The model under review builds one solid part; all positions refer to its coordinate system, in mm. Face numbers are marked on the shaded views. A direction names the side the tool comes from. Give positions to 0.01 mm unless a question says otherwise; leave off trailing zeros. Write each loop counter-clockwise with the first axis right and the second up, starting at its lowest first coordinate (ties: lowest second). Pieces come first, ordered by that corner, then holes. Notation, with made-up numbers: (18.5, -14) -> (65.5, -14) arc R13 cw to (65.5, -3) -> close; hole circle Ø6 at (53, 58). An arc over 180 degrees is marked (long way). Use CSV: the item, a comma, the result in double quotes.
```python
from build123d import *

# Parameters (mm, degrees)
SKETCH_W        = 37
SKETCH_H        = 32
PAD_DEPTH       = 4
SKETCH001_W     = 4
SKETCH001_H     = 32
PAD001_DEPTH    = 10
SKETCH002_R     = 1.4
POCKET_DEPTH    = 100
POCKET003_DEPTH = 100
SKETCH004_R     = 1.3
SKETCH004_R_2   = 4.5
POCKET007_DEPTH = 5
SKETCH008_R     = 1.8
POCKET009_DEPTH = 10
CHAMFER_SIZE    = 1
CHAMFER001_SIZE = 0.2


with BuildPart() as part:
    # Sketch → Pad (new body)
    with BuildSketch(Plane.XY):
        Rectangle(SKETCH_W, SKETCH_H)
    extrude(amount=PAD_DEPTH)

    # Sketch001 (on Face6 of Pad) → Pad001 (join)
    with BuildSketch(Plane.XY.offset(4)):
        with Locations((16.5, 0)):
            Rectangle(SKETCH001_W, SKETCH001_H)
        with Locations((-16.5, 0)):
            Rectangle(SKETCH001_W, SKETCH001_H)
    extrude(amount=PAD001_DEPTH)

    # Sketch002 (on Face13 of Pad001) → Pocket (cut)
    with BuildSketch(Plane.YZ.offset(18.5)):
        with Locations((-11, 11)):
            Circle(SKETCH002_R)
        with Locations((11, 11)):
            Circle(SKETCH002_R)
    extrude(amount=-POCKET_DEPTH, mode=Mode.SUBTRACT)

    # Sketch006 → Pocket003 (cut)
    with BuildSketch(Plane(origin=(-20, 0, 0), x_dir=(0, -1, 0), z_dir=(-1, 0, 0))):
        with BuildLine():
            ThreePointArc((8, 10.650166), (0, 29.2), (-8, 10.650166))
            Line((-8, 10.650166), (-8, 7.2))
            Line((-8, 7.2), (8, 7.2))
            Line((8, 7.2), (8, 10.650166))
        make_face()
    extrude(amount=-POCKET003_DEPTH, mode=Mode.SUBTRACT)

    # Sketch004 → Pocket007 (cut)
    with BuildSketch(Plane.XY.offset(4)):
        with Locations((0, 8)):
            Circle(SKETCH004_R)
        with Locations((8, 0)):
            Circle(SKETCH004_R)
        with Locations((0, -8)):
            Circle(SKETCH004_R)
        with Locations((-8, 0)):
            Circle(SKETCH004_R)
        Circle(SKETCH004_R_2)
        with Locations((5.656854, 5.656854)):
            Circle(SKETCH004_R)
        with Locations((-5.656854, 5.656854)):
            Circle(SKETCH004_R)
        with Locations((-5.656854, -5.656854)):
            Circle(SKETCH004_R)
        with Locations((5.656854, -5.656854)):
            Circle(SKETCH004_R)
    extrude(amount=-POCKET007_DEPTH, mode=Mode.SUBTRACT)

    # Sketch008 → Pocket009 (cut)
    with BuildSketch(Plane(origin=(0, 0, 0), x_dir=(1, 0, 0), z_dir=(0, 0, -1))):
        with Locations((10, 10)):
            Circle(SKETCH008_R)
        with Locations((-10, 10)):
            Circle(SKETCH008_R)
        with Locations((-10, -10)):
            Circle(SKETCH008_R)
        with Locations((10, -10)):
            Circle(SKETCH008_R)
    extrude(amount=-POCKET009_DEPTH, mode=Mode.SUBTRACT)

    # Chamfer
    chamfer_edges = [part.edges().sort_by_distance(p)[0] for p in [
        (-6.956854, -5.656854, 4),
        (-1.3, -8, 4),
        (4.356854, -5.656854, 4),
        (6.7, 0, 4),
        (4.356854, 5.656854, 4),
        (-1.3, 8, 4),
        (-6.956854, 5.656854, 4),
        (-9.3, 0, 4),
    ]]
    chamfer(chamfer_edges, length=CHAMFER_SIZE)

    # Chamfer001
    chamfer001_edges = [part.edges().sort_by_distance(p)[0] for p in [
        (-6.956854, -5.656854, 0),
        (-9.3, 0, 0),
        (-6.956854, 5.656854, 0),
        (-1.3, 8, 0),
        (4.356854, 5.656854, 0),
        (6.7, 0, 0),
        (4.356854, -5.656854, 0),
        (-1.3, -8, 0),
        (-11.8, -10, 0),
        (-11.8, 10, 0),
        (8.2, 10, 0),
        (8.2, -10, 0),
    ]]
    chamfer(chamfer001_edges, length=CHAMFER001_SIZE)


solid = part.part
```
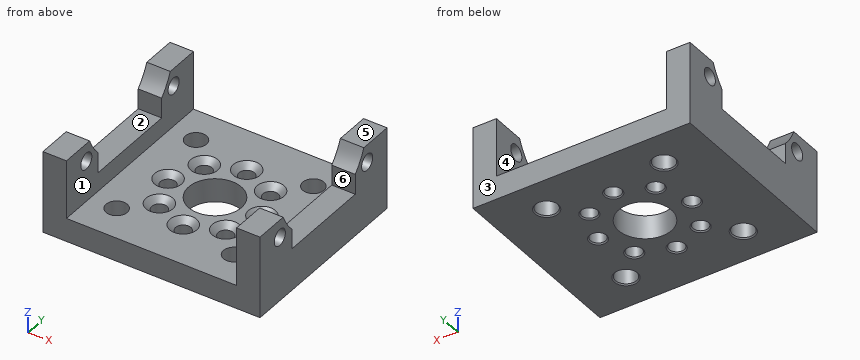
Q1. The part is to be moulded in two halves that separate along Y. For the marked faces 1, 2 and 3, say which applies: pulls with the +Y half, pulls with the -Y half, needs draft (parallel to the pull), parting line crosses it, or undercut.
Derived:
face 1,"needs draft"
face 2,"undercut"
face 3,"pulls with the +Y half"
Q2. Consider section B-B (x = 0). Write out the cut boundary in (y, z), then the cut area to 3 significant figures.
Derived:
outline,"(-16, 0) -> (-9.5, 0) -> (-9.3, 0.2) -> (-9.3, 3) -> (-10.3, 4) -> (-16, 4) -> close; (-6.7, 0.2) -> (-6.5, 0) -> (-4.5, 0) -> (-4.5, 4) -> (-5.7, 4) -> (-6.7, 3) -> close; (4.5, 0) -> (6.5, 0) -> (6.7, 0.2) -> (6.7, 3) -> (5.7, 4) -> (4.5, 4) -> close; (9.3, 0.2) -> (9.5, 0) -> (16, 0) -> (16, 4) -> (10.3, 4) -> (9.3, 3) -> close"
area,"69.1 mm2"
Q3. Machinability: for the marked faces 4, 5 and 6, which of the approach directions +Z, -Z, +X, -X, +Y, -Y give a long, thin tool a straight path to every point of the face, cutting with its end or side? Answer none if there is none.
Derived:
face 4,"+Z, +Y, -Y"
face 5,"+Z, +X, -X, +Y, -Y"
face 6,"+Z, +X, -X"
Q4. Insertion check: pin 1 (3.5 mm diameter, centred on x = -5.66, y = -5.66, fed in from -Z); pin 2 (4 mm diameter, centred on x = -10, y = -10, fed in from +Z); pin 3 (2 mm diameter, centred on x = -8, y = 0, fed in from -Z); pin 4 (3 mm diameter, centred on x = 0, y = 8, fed in from +Z). Each pin has a flat end and moves straight along its axis. Give the tip position at first contact, or say it passes through.
Derived:
pin 1,"stops at z = 0"
pin 2,"stops at z = 4"
pin 3,"passes through"
pin 4,"stops at z = 3.2"
Q5. Consider section C-C (z = 2). State how many separate pieces and enclosed holes the cut face has, then the cut area to 3 significant figures.
Derived:
separate pieces,"1"
enclosed holes,"13"
area,"1,040 mm2"
Q6. To check wall thickness, follow probe 1 along X at (y, z) = (-10, 3.2); probe 2 along X at (y, z) = (-14, 8.5); probe 3 along Y at (x, z) = (1, 3.5). State the ranges of each line that lie inside material, in increasing order.
Derived:
probe 1,"x = -18.5 to -11.8, -8.2 to 8.2, 11.8 to 18.5"
probe 2,"x = -18.5 to -14.5, 14.5 to 18.5"
probe 3,"y = -16 to -9.5, -6.5 to -4.39, 4.39 to 6.5, 9.5 to 16"
Q7. Consider section A-A (y = 0). Write out the cut boundary in (x, z).
Derived:
outline,"(-18.5, 0) -> (-9.5, 0) -> (-9.3, 0.2) -> (-9.3, 3) -> (-10.3, 4) -> (-14.5, 4) -> (-14.5, 7.2) -> (-18.5, 7.2) -> close; (-6.7, 0.2) -> (-6.5, 0) -> (-4.5, 0) -> (-4.5, 4) -> (-5.7, 4) -> (-6.7, 3) -> close; (4.5, 0) -> (6.5, 0) -> (6.7, 0.2) -> (6.7, 3) -> (5.7, 4) -> (4.5, 4) -> close; (9.3, 0.2) -> (9.5, 0) -> (18.5, 0) -> (18.5, 7.2) -> (14.5, 7.2) -> (14.5, 4) -> (10.3, 4) -> (9.3, 3) -> close"
